Work out the finished part from the listing and answer in its coordinate system (mm). Face numbers are marked on the shaded views. A direction names the side the tool comes from. Round coordinates to 2 decimals unless told otherwise and drop trailing zeros. Loops run counter-clockwise (first coordinate to the right, second up) from the corner with the lowest first, then second, coordinate; pieces in that order, holes last. Notation, with made-up numbers: (8, 29) -> (38, 29) arc R7 cw to (38, 37) -> close; hole circle Ø6 at (23.5, 11.25). An arc over 180 degrees is marked (long way). Use one line per item in the form item = value.
```python
from build123d import *

# Parameters (mm, degrees)
SKETCH_1_R          = 25
SKETCH_1_R_2        = 16.5
EXTRUDE_1_DEPTH     = 3
SKETCH_2_R          = 19
CUT_EXTRUDE_1_DEPTH = 1.5
CUT_EXTRUDE_2_DEPTH = 1.5
SKETCH_4_R          = 1
CUT_EXTRUDE_3_DEPTH = 31.5
SKETCH_6_R          = 1.5
CUT_EXTRUDE_4_DEPTH = 1


with BuildPart() as part:
    # 草图1 → 凸台-拉伸1 (new body)
    with BuildSketch(Plane.XY):
        Circle(SKETCH_1_R)
        Circle(SKETCH_1_R_2, mode=Mode.SUBTRACT)
    extrude(amount=EXTRUDE_1_DEPTH)

    # 草图2 → 切除-拉伸1 (cut)
    with BuildSketch(Plane.XY.offset(3)):
        Circle(SKETCH_2_R)
    extrude(amount=-CUT_EXTRUDE_1_DEPTH, mode=Mode.SUBTRACT)

    # 草图3 → 切除-拉伸2 (cut)
    with BuildSketch(Plane.XY.offset(3)):
        Polygon((0, -29.98623759), (8, -29.98623759), (8, -6.378834071), (-8, -6.378834071), (-8, -29.98623759), align=None)
    extrude(amount=-CUT_EXTRUDE_2_DEPTH, mode=Mode.SUBTRACT)

    # 草图4 → 切除-拉伸3 (cut)
    with BuildSketch(Plane.XY.offset(3)):
        with Locations((0, 20.5)):
            Circle(SKETCH_4_R)
        with Locations((17.753520778, -10.25)):
            Circle(SKETCH_4_R)
        with Locations((-17.753520778, -10.25)):
            Circle(SKETCH_4_R)
    extrude(amount=-CUT_EXTRUDE_3_DEPTH, mode=Mode.SUBTRACT)

    # 草图6 → 切除-拉伸4 (cut)
    with BuildSketch(Plane(origin=(0, 0, 0), x_dir=(-1, 0, 0), z_dir=(0, 0, -1))):
        with Locations((0, 20.5)):
            Circle(SKETCH_6_R)
        with Locations((17.753520778, -10.25)):
            Circle(SKETCH_6_R)
        with Locations((-17.753520778, -10.25)):
            Circle(SKETCH_6_R)
    extrude(amount=-CUT_EXTRUDE_4_DEPTH, mode=Mode.SUBTRACT)

    # 草图8 → 切除-旋转1 (revolve, cut)
    with BuildSketch(Plane(origin=(0, 0, 0), x_dir=(1, 0, 0), z_dir=(0, 1, 0))):
        Polygon((-22.5, -1), (-22.5, -3), (-22.5, -4.221155356), (-26.330731104, -4.221155356), (-26.330731104, -3), (-26.330731104, 1.037990449), (-24, 1.037990449), (-23.5, 1.037990449), (-23.5, 0), align=None)
    revolve(axis=Axis((0, 0, 0), (0, 0, 1)), mode=Mode.SUBTRACT)


solid = part.part
```
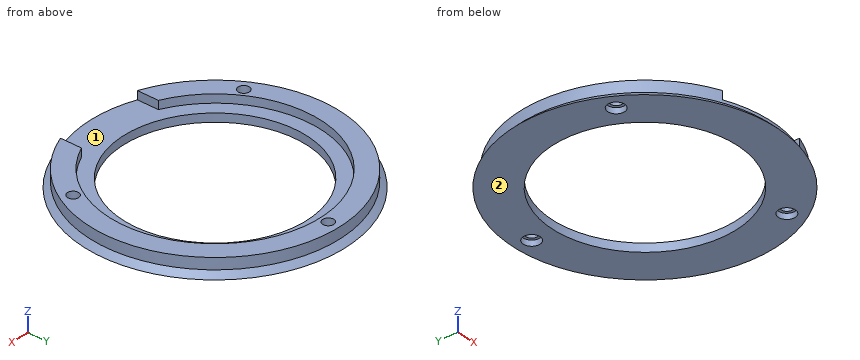
(1) Given P1, Ø0.9, axis at x = -0.5, y = 20, coming from the -Z side; P2, Ø1.6, axis at x = -17.75, y = -10.25, coming from the -Z side (3 decimals); P3, Ø5, axis at x = 17.75, y = -10.25, coming from the +Z side; P4, Ø1.6, axis at y = -19, z = 2.5, coming from the +X side, each flat-ended and moving along its own axis, determine where each tip first touches the part or whether it passes through.
Completed:
P1 = 1
P2 = through
P3 = 3
P4 = 13.23
(2) For the marked faces 1 and 2, determine the directions among +Z, -Z, +X, -X, +Y, -Y from which every point of the face is accessible in a straight line to the end or side of a thin tool.
Completed:
face_1 = +Z
face_2 = -Z, +X, -X, +Y, -Y
(3) Find section B-B, the plane x = 0. Write down the section's boundary in (y, z), then the cut area to 4 significant figures.
Completed:
outline = (-23.5, 0) -> (-16.5, 0) -> (-16.5, 1.5) -> (-22.5, 1.5) -> (-22.5, 1) -> close; (16.5, 0) -> (19, 0) -> (19, 1) -> (19.5, 1) -> (19.5, 3) -> (19, 3) -> (19, 1.5) -> (16.5, 1.5) -> close; (21.5, 1) -> (22, 1) -> (22, 0) -> (23.5, 0) -> (22.5, 1) -> (22.5, 3) -> (21.5, 3) -> close
area = 17.25 mm2
(4) Find section C-C, the plane z = 2.05. Write down the section's boundary in (x, y), then the cut area to 3 significant figures.
Completed:
outline = (-8, -21.03) -> (-8, -17.23) arc R19 cw (long way) to (8, -17.23) -> (8, -21.03) arc R22.5 ccw (long way) to start; hole circle Ø2 at (-17.75, -10.25); hole circle Ø2 at (0, 20.5); hole circle Ø2 at (17.75, -10.25)
area = 389 mm2
(5) Consider L1, parallel to Y at x = 0, z = 0.75; L2, parallel to Z at x = -4.5, y = -17; L3, parallel to X at y = -7, z = 2.6. Determine where each line is inside the solid, lowest interval first.
Completed:
L1 = -22.75 to -16.5, 16.5 to 19, 22 to 22.75
L2 = 0 to 1.5
L3 = -21.38 to -17.66, 17.66 to 21.38
(6) Find section A-A, the plane y = 0. Write down the section's boundary in (x, z).
Completed:
outline = (-23.5, 0) -> (-16.5, 0) -> (-16.5, 1.5) -> (-19, 1.5) -> (-19, 3) -> (-22.5, 3) -> (-22.5, 1) -> close; (16.5, 0) -> (23.5, 0) -> (22.5, 1) -> (22.5, 3) -> (19, 3) -> (19, 1.5) -> (16.5, 1.5) -> close
(7) Find section D-D, the plane y = -10.25. State how many separate pieces and enclosed holes the cut face has, then the cut area to 3 significant figures.
Completed:
separate_pieces = 4
enclosed_holes = 0
area = 20.5 mm2
